Read the model definition and answer for the solid it produces. Units are mm, in the model's axes. A direction names the side the tool comes from. Coordinates: 2 decimals unless noted, no trailing zeros. Write each loop counter-clockwise with the first axis right and the second up, starting at its lowest first coordinate (ties: lowest second). Pieces come first, ordered by that corner, then holes.
Item 1: Section D-D (x = 45) is taken. Give the vertices of the cut face in (y, z), then the cut area to 3 significant figures.
Item 2: Section A-A (y = 2.75) is taken. Give the vertices of the cut face in (x, z), then the cut area to 3 significant figures.
Item 3: A tool of negligible diameter and unlimited length cuts with its end or side. For faces 1 (the face through (10.598, 8, 1)), 2 (the face through (40, 9.265, 1)), 3 (the face through (38.379, -4, 1)), from which of +Z, -Z, +X, -X, +Y, -Y can it reach the whole face along a straight path? Write none if from no direction.
Item 4: Each of these flat-tipped pins is pushed along its axis until it touches: P1, Ø0.5, axis at x = 34, z = 1, coming from the -Y side; P2, Ø4, axis at x = 47, y = 2.5, coming from the -Z side; P3, Ø0.8, axis at x = 31.5, z = 0.5, coming from the +Y side. Where does it stop, or does it pass through?
Item 5: Determine the mould class of faces 4 (the face through (13.773, 8, 1)), 5 (the face through (59.017, 2, 1)), 6 (the face through (9, 9.265, 1)) for opening direction X: released by +X, released by -X, zero draft, split by the parting line, or undercut.
Item 6: Straight lines are drawn through the part: probe 1 along X at (y, z) = (2, 0.5); probe 2 along Y at (x, z) = (27.5, 1.15); probe 3 along X at (y, z) = (3, 1.1). For each, find the intervals that lie inside material, in ascending order.
Item 7: Section B-B (z = 0.95) is taken. Give the vertices of the cut face in (x, y) (1 decimal).
Item 8: Section C-C (x = 33.5) is taken. Give the vertices of the cut face in (y, z).
Autodesk Inventor part; units mm, degrees
ref_plane "YZ Plane" through (0, 0, 0) normal (1, 0, 0) x (0, 1, 0)
ref_plane "XZ Plane" through (0, 0, 0) normal (0, 1, 0) x (-1, 0, 0)
ref_plane "XY Plane" through (0, 0, 0) normal (0, 0, 1) x (1, 0, 0)
sketch "Sketch1" plane through (0, 0, 0) normal (0, 0, 1) x (1, 0, 0)
  line L0 (8.2169, 9.2649) -> (8.2169, -5.0211)
  line L1 (8.2169, -5.0211) -> (41.5544, -5.0211)
  line L2 (41.5544, -5.0211) -> (59.0169, -1.8469)
  line L3 (59.0169, -1.8469) -> (59.0169, 6.0906)
  line L4 (59.0169, 6.0906) -> (41.5544, 9.2649)
  line L5 (41.5544, 9.2649) -> (8.2169, 9.2649)
  line L6 (59.0169, 2.1219) -> (8.2169, 2.1219) construction
  line L7 (3.1369, 0) -> (74.2569, 0)
  line L8 (0, 13.5507) -> (0, -6.4497)
  dimension "d1" = 33.3375
  dimension "d2" = 50.8
  dimension "d3" = 7.9375
  dimension "d92" = 7.143
  dimension "d93" = 2.1218
  dimension "d94" = 8.2169
extrude "Extrusion1" add sketch "Sketch1" along normal blind 1.5875
sketch "Sketch12" plane through (0, 0, 1.5875) normal (0, 0, 1) x (1, 0, 0)
  line L0 (8.2169, 9.2649) -> (41.5544, 9.2649)
  line L1 (8.2169, -5.0211) -> (8.2169, 9.2649)
  line L2 (22.5044, 9.2649) -> (38.3794, 9.2649)
  line L3 (38.3794, 9.2649) -> (38.3794, 7.6774)
  line L4 (38.3794, 7.6774) -> (22.5044, 7.6774)
  line L5 (22.5044, 7.6774) -> (22.5044, 9.2649)
  dimension "d63" = 15.875
  dimension "d64" = 1.5875
  dimension "d65" = 14.2875
extrude "Extrusion12" cut sketch "Sketch12" against normal through all
sketch "Sketch13" plane through (0, 0, 1.5875) normal (0, 0, 1) x (1, 0, 0)
  line L0 (8.2169, 9.2649) -> (22.5044, 9.2649)
  line L1 (38.3794, 7.6774) -> (22.5044, 7.6774)
  line L2 (10.5981, 9.2649) -> (10.5981, 7.6774)
  arc A0 (10.5981, 7.6774) -> (13.7731, 7.6774) centre (12.1856, 7.6774) ccw
  line L3 (13.7731, 7.6774) -> (13.7731, 9.2649)
  line L4 (22.5044, 7.6774) -> (22.5044, 9.2649)
  line L5 (8.2169, -5.0211) -> (8.2169, 9.2649)
  line L6 (41.5544, -5.0211) -> (8.2169, -5.0211)
  line L7 (59.0169, -1.8469) -> (41.5544, -5.0211)
  line L8 (59.0169, 6.0906) -> (59.0169, -1.8469)
  line L9 (41.5544, 9.2649) -> (59.0169, 6.0906)
  line L10 (38.3794, 9.2649) -> (41.5544, 9.2649)
  line L11 (38.3794, 9.2649) -> (38.3794, 7.6774)
  dimension "d68" = 1.5875
  dimension "d69" = 1.5875
  dimension "d70" = 3.9688
extrude "Extrusion13" cut sketch "Sketch13" against normal blind 25.4 contours L0 L3 A0 L2
ref_plane "Work Plane5" through (22.5044, 2.1211, 1.5875) normal (0, 1, 0) x (1, 0, 0)
mirror "Mirror2" about plane through (22.5044, 2.1211, 1.5875) normal (0, 1, 0) of "Extrusion12", "Extrusion13"
sketch "Sketch14" plane through (0, 0, 1.5875) normal (0, 0, 1) x (1, 0, 0)
  line L0 (3.1369, 2.1211) -> (74.2569, 2.1211)
  line L1 (13.7731, 9.2649) -> (22.5044, 9.2649)
  line L2 (8.2169, -5.0211) -> (8.2169, 9.2649)
  point P0 (53.4606, 2.1219)
  dimension "d95" = 45.2437
  dimension "d96" = 7.143
hole "Hole1" at (53.4606, 2.1219, 1.5875) direction (0, 0, -1) diameter 3.175 end through all
sketch "Sketch15" plane through (0, 0, 1.5875) normal (0, 0, 1) x (1, 0, 0)
  line L0 (10.5981, -5.0211) -> (10.5981, -3.4351)
  line L1 (59.0169, 6.0906) -> (57.4294, 4.5031)
  line L2 (57.4294, 4.5031) -> (57.4294, -0.2594)
  line L3 (57.4294, -0.2594) -> (59.0169, -1.8469)
  dimension "d82" = 4.7625
  dimension "d84" = 1.5875
hole "Hole2" at (57.4294, 4.5031, 1.5875) at (57.4294, -0.2594, 1.5875) direction (0, 0, -1) diameter 0.762 end through all
properties part number "pcb"
Established:
1. outline: (-4.39, 0) - (8.64, 0) - (8.64, 1.59) - (-4.39, 1.59) - close
1. area: 20.7 mm2
2. outline: (8.22, 0) - (52, 0) - (52, 1.59) - (8.22, 1.59) - close; (54.92, 0) - (59.02, 0) - (59.02, 1.59) - (54.92, 1.59) - close
2. area: 76.0 mm2
3. face 1: +Z, -Z, +Y
3. face 2: +Z, -Z, +X, -X, +Y
3. face 3: +Z, -Z, -Y
4. P1: stops at y = -3.44
4. P2: stops at z = 0
4. P3: stops at y = 7.68
5. face 4: undercut
5. face 5: released by +X
5. face 6: zero draft
6. probe 1: x = 8.22 to 51.88, 55.04 to 59.02
6. probe 2: y = -3.44 to 7.68
6. probe 3: x = 8.22 to 52.14, 54.78 to 59.02
7. outline: (8.2, -5) - (10.6, -5) - (10.6, -3.4) arc R1.6 cw to (13.8, -3.4) - (13.8, -5) - (22.5, -5) - (22.5, -3.4) - (38.4, -3.4) - (38.4, -5) - (41.6, -5) - (59, -1.8) - (59, 6.1) - (41.6, 9.3) - (38.4, 9.3) - (38.4, 7.7) - (22.5, 7.7) - (22.5, 9.3) - (13.8, 9.3) - (13.8, 7.7) arc R1.6 cw to (10.6, 7.7) - (10.6, 9.3) - (8.2, 9.3) - close; hole circle Ø3.2 at (53.5, 2.1); hole circle Ø0.8 at (57.4, -0.3); hole circle Ø0.8 at (57.4, 4.5)
8. outline: (-3.44, 0) - (7.68, 0) - (7.68, 1.59) - (-3.44, 1.59) - close
